from build123d import *

# Parameters (mm, degrees)
SKETCH1_R               = 25
BOSS_EXTRUDE1_DEPTH     = 2.5
SKETCH3_W               = 50
SKETCH3_H               = 190
BOSS_EXTRUDE2_DEPTH     = 2.5
SKETCH4_W               = 10
SKETCH4_H               = 60
BOSS_EXTRUDE3_DEPTH     = 2.5
CUT_EXTRUDE2_DEPTH      = 164.802472509
CUT_EXTRUDE2_DEPTH_BACK = 164.802472509
SKETCH7_R               = 11
SKETCH7_R_2             = 12.7
FILLET1_R               = 5


with BuildPart() as part:
    # Sketch1 → Boss-Extrude1 (new, symmetric)
    with BuildSketch(Plane.XY):
        with Locations((0, -30)):
            Circle(SKETCH1_R)
    extrude(amount=BOSS_EXTRUDE1_DEPTH, both=True)

    # Sketch3 → Boss-Extrude2 (add, symmetric)
    with BuildSketch(Plane.XY):
        with Locations((0, 65)):
            Rectangle(SKETCH3_W, SKETCH3_H)
    extrude(amount=BOSS_EXTRUDE2_DEPTH, both=True)

    # Sketch4 → Boss-Extrude3 (add, symmetric)
    with BuildSketch(Plane.XY):
        with Locations((30, 130)):
            Rectangle(SKETCH4_W, SKETCH4_H)
    extrude(amount=BOSS_EXTRUDE3_DEPTH, both=True)

    # Sketch7 → Cut-Extrude2 (cut, two sides: drawn at the far end of the back side and taken through both)
    with BuildSketch(Plane.XY.offset(-CUT_EXTRUDE2_DEPTH_BACK)):
        Circle(SKETCH7_R)
        with Locations((0, -30)):
            Circle(SKETCH7_R_2)
    extrude(amount=CUT_EXTRUDE2_DEPTH + CUT_EXTRUDE2_DEPTH_BACK, mode=Mode.SUBTRACT)

    # Fillet1
    fillet1_edges = [part.edges().sort_by_distance(p)[0] for p in [
        (25, 100, 0),
    ]]
    fillet(fillet1_edges, radius=FILLET1_R)


solid = part.part
Here's how the part is built. I have some questions about the finished solid (model axes, mm). A direction names the side the tool comes from. Round coordinates to 2 decimals unless told otherwise and drop trailing zeros. Order: outer loops, then holes, each group sorted by start corner. A loop starts at its lowest first (then second) coordinate and runs counter-clockwise, first axis right, second up. Notation, with made-up numbers: M 87,-33.5 L 93,-33.5 A22 cw 93,-16.5 Z; hole C 77,-28.75 d10. An arc over 180 degrees is marked long. Return JSON: item names as keys, results as strings. Group by question number.
1. If we section it at D-D on y = 64: List the corners of the cut face in (x, z) for me, then the cut area to 3 significant figures.
2. If we section it at B-B on z = -0.2: List the corners of the cut face in (x, y) for me, then the cut area to 3 significant figures.
3. Please list where these lines run through material, in increasing order: probe 1 along Y at (x, z) = (0, 1.3); probe 2 along X at (y, z) = (0, 0.15); probe 3 along Y at (x, z) = (9, -0.9).
4. I'm going to push flat-ended pins straight in: pin 1 Ø1.5 at (y, z) = (38, 1) entering from +X; pin 2 Ø2 at (x, z) = (4, 0) entering from -Y. Where does each tip first touch, or does it pass through?
5. If we section it at A-A on y = 0: List the corners of the cut face in (x, z) for me.
6. If we section it at C-C on x = 0: List the corners of the cut face in (y, z) for me, then the cut area to 3 significant figures.
7. If we mould it in two halves opening along Y, with no side actions, what happens to faces 3 (the face through (-25, 64, 0)), 4 (the face through (5.86, -41.267, -0.035)), 5 (the face through (5, 160, 0))? For each: pulls with the +Y half, pulls with the -Y half, needs draft (parallel to the pull), parting line crosses it, or undercut.
8. On a 3-axis mill with a long thin cutter (end or side, diameter ignored), from which of +Z, -Z, +X, -X, +Y, -Y can I reach the whole of each face in a straight line? I mean faces 1 (the face through (35, 130, 0)), 2 (the face through (25, 32, 0)). Say none if no direction works.
Reply:
{
 "1": {"outline": "M -25,-2.5 L 25,-2.5 L 25,2.5 L -25,2.5 Z", "area": "250 mm^2"},
 "2": {"outline": "M -25,-30 A25 ccw 25,-30 L 25,95 A5 cw 30,100 L 35,100 L 35,160 L -25,160 Z; hole C 0,-30 d25.4; hole C 0,0 d22", "area": "10,200 mm^2"},
 "3": {"probe 1": "-55 to -42.7, -17.3 to -11, 11 to 160", "probe 2": "-25 to -11, 11 to 25", "probe 3": "-53.32 to -38.96, -21.04 to -6.32, 6.32 to 160"},
 "4": {"pin 1": "x = 25", "pin 2": "y = -54.82"},
 "5": {"outline": "M -25,-2.5 L -11,-2.5 L -11,2.5 L -25,2.5 Z; M 11,-2.5 L 25,-2.5 L 25,2.5 L 11,2.5 Z"},
 "6": {"outline": "M -55,-2.5 L -42.7,-2.5 L -42.7,2.5 L -55,2.5 Z; M -17.3,-2.5 L -11,-2.5 L -11,2.5 L -17.3,2.5 Z; M 11,-2.5 L 160,-2.5 L 160,2.5 L 11,2.5 Z", "area": "838 mm^2"},
 "7": {"face 3": "needs draft", "face 4": "undercut", "face 5": "pulls with the +Y half"},
 "8": {"face 1": "+Z, -Z, +X, +Y, -Y", "face 2": "+Z, -Z, +X, -Y"}
}
